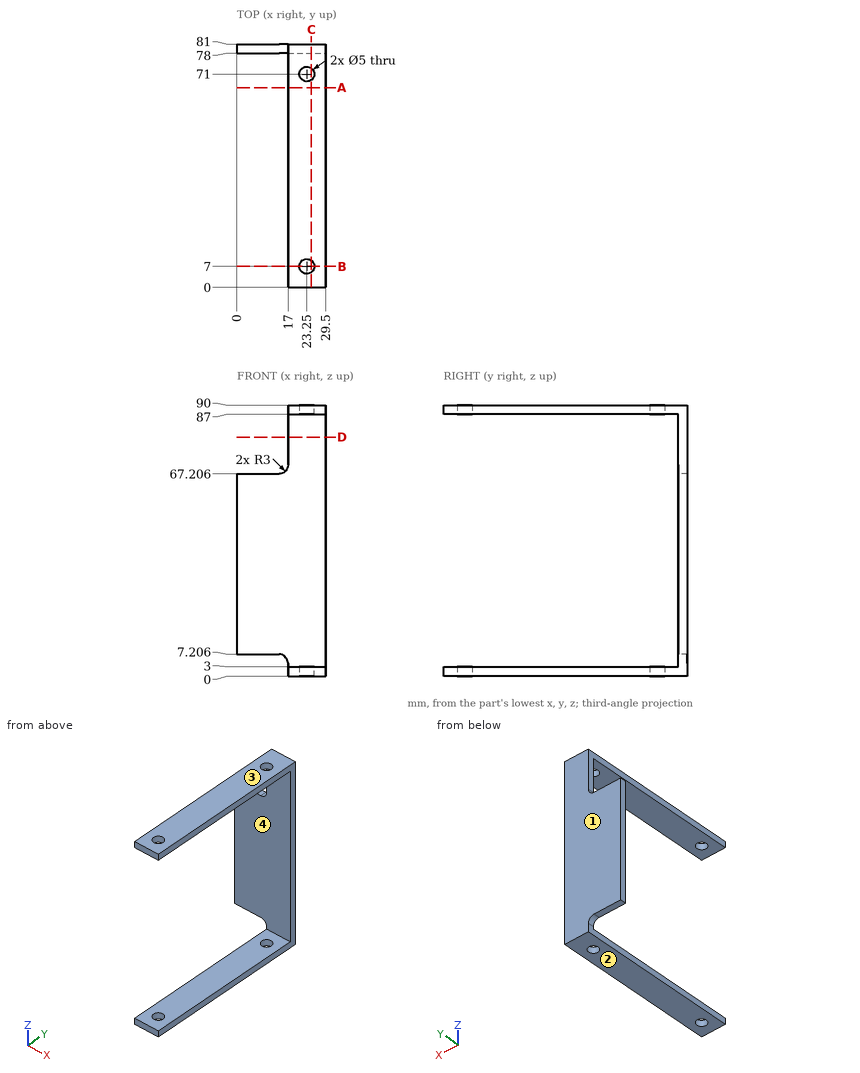
Answer from the drawing. Dimensions are ordinates in mm from the lowest x, y and z of the part. Round coordinates to 2 decimals unless told otherwise and drop trailing zeros. Order: outer loops, then holes, each group sorted by start corner. A loop starts at its lowest first (then second) coordinate and runs counter-clockwise, first axis right, second up.
1) Flat-ended cylindrical pins translate along their axes: pin 1 (0.9 mm diameter, centred on x = 9, y = 79, fed in from -Z); pin 2 (4.5 mm diameter, centred on y = 31.5, z = 1.5, fed in from -X); pin 3 (15 mm diameter, centred on x = 17, z = 25.5, fed in from -Y). Find the tip coordinate at first contact, or state that the pin passes through.
2) The part is cut by section C-C on x = 24.75. Write down the section's boundary in (y, z).
3) The mould has two halves that part along Z. Classify the marked faces 1, 2, 3 and 4: released by +Z, released by -Z, zero draft, split by the parting line, or undercut.
4) The part is cut by section A-A on y = 66.5. Write down the section's boundary in (x, z), plus the area to 3 significant figures.
5) The part is cut by section B-B on y = 7. Write down the section's boundary in (x, z), plus the area to 3 significant figures.
6) Straight lines are drawn through the part: L1, parallel to Y at x = 23.25, z = 1.15; L2, parallel to Z at x = 19.5, y = 77; L3, parallel to X at y = 7, z = 88.7. For each, find the intervals that lie inside material, in ascending order.
7) The part is cut by section D-D on z = 79.5. Write down the section's boundary in (x, y), plus the area to 3 significant figures.
Resolved:
1. pin 1: stops at z = 7.21
1. pin 2: stops at x = 17
1. pin 3: stops at y = 78
2. outline: (0, 0) - (5, 0) - (5, 3) - (0, 3) - close; (0, 87) - (5, 87) - (5, 90) - (0, 90) - close; (9, 0) - (69, 0) - (69, 3) - (9, 3) - close; (9, 87) - (69, 87) - (69, 90) - (9, 90) - close; (73, 0) - (81, 0) - (81, 90) - (73, 90) - (73, 87) - (78, 87) - (78, 3) - (73, 3) - close
3. face 1: zero draft
3. face 2: released by -Z
3. face 3: released by +Z
3. face 4: undercut
4. outline: (17, 0) - (29.5, 0) - (29.5, 3) - (17, 3) - close; (17, 87) - (29.5, 87) - (29.5, 90) - (17, 90) - close
4. area: 75.0 mm2
5. outline: (17, 0) - (20.75, 0) - (20.75, 3) - (17, 3) - close; (17, 87) - (20.75, 87) - (20.75, 90) - (17, 90) - close; (25.75, 0) - (29.5, 0) - (29.5, 3) - (25.75, 3) - close; (25.75, 87) - (29.5, 87) - (29.5, 90) - (25.75, 90) - close
5. area: 45.0 mm2
6. L1: y = 0 to 4.5, 9.5 to 68.5, 73.5 to 81
6. L2: z = 0 to 3, 87 to 90
6. L3: x = 17 to 20.75, 25.75 to 29.5
7. outline: (17, 78) - (29.5, 78) - (29.5, 81) - (17, 81) - close
7. area: 37.5 mm2
